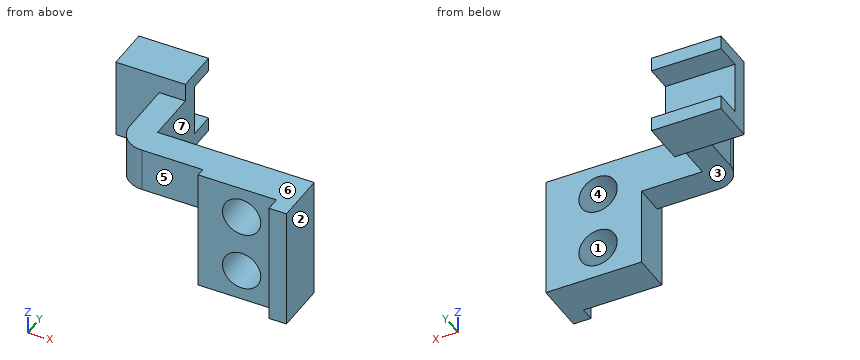
Autodesk Inventor part; units mm, degrees
ref_plane "YZ Plane" through (0, 0, 0) normal (1, 0, 0) x (0, 1, 0)
ref_plane "XZ Plane" through (0, 0, 0) normal (0, 1, 0) x (-1, 0, 0)
ref_plane "XY Plane" through (0, 0, 0) normal (0, 0, 1) x (1, 0, 0)
sketch "Sketch1" plane through (0, 0, 0) normal (0, 0, 1) x (1, 0, 0)
  line L0 (0, 0) -> (-100, 0)
  line L1 (-100, 0) -> (-100, 80)
  line L2 (-100, 80) -> (-550, 80)
  line L3 (-550, 80) -> (-550, 130)
  line L4 (-550, 130) -> (-1050, 130)
  line L5 (-1050, 130) -> (-1050, 600)
  line L6 (-1050, 600) -> (-900, 600)
  line L7 (-900, 600) -> (-900, 300)
  line L8 (-900, 300) -> (0, 300)
  line L9 (0, 300) -> (0, 0)
  line L10 (-550, 130) -> (-550, 300)
  dimension "d0" = 100
  dimension "d1" = 80
  dimension "d2" = 450
  dimension "d3" = 50
  dimension "d4" = 500
  dimension "d5" = 470
  dimension "d6" = 150
  dimension "d7" = 300
extrude "Extrusion1" add sketch "Sketch1" against normal blind 700 contours L0 L1 L2 L3 L10 L8 L9
sketch "Sketch2" plane through (0, 0, 0) normal (0, 0, 1) x (1, 0, 0)
  line L0 (-100, 80) -> (-550, 80) construction
  line L1 (-550, 80) -> (-550, 130)
  line L2 (-550, 80) -> (-550, 300) construction
  line L3 (-550, 130) -> (-1050, 130)
  line L4 (-1050, 130) -> (-1050, 600)
  line L5 (-1050, 600) -> (-900, 600)
  line L6 (-900, 600) -> (-900, 300)
  line L7 (-900, 300) -> (-550, 300)
  line L8 (-550, 300) -> (-550, 80) construction
  line L9 (-550, 130) -> (-550, 300)
  point P0 (0, 0)
  dimension "d10" = 50
  dimension "d11" = 500
  dimension "d12" = 470
  dimension "d13" = 150
  dimension "d14" = 300
extrude "Extrusion2" add sketch "Sketch2" against normal blind 250
sketch "Sketch3" plane through (-900, 300, 0) normal (1, 0, 0) x (0, 0, -1)
  line L0 (0, 300) -> (250, 300) construction
  line L1 (0, 300) -> (-105, 300)
  line L2 (-105, 300) -> (-105, 550)
  line L3 (-105, 550) -> (-25, 550)
  line L4 (-25, 550) -> (-25, 400)
  line L5 (-25, 400) -> (275, 400)
  line L6 (275, 400) -> (275, 550)
  line L7 (275, 550) -> (355, 550)
  line L8 (355, 550) -> (355, 300)
  line L9 (355, 300) -> (0, 300)
  point P0 (0, -300)
  dimension "d17" = 105
  dimension "d18" = 250
  dimension "d19" = 80
  dimension "d20" = 150
  dimension "d21" = 300
  dimension "d22" = 80
extrude "Extrusion3" add sketch "Sketch3" against normal blind 400
fillet "Fillet1" radius 150 1 edges at (-1050, 130, -125)
sketch "Sketch4" plane through (-550, 300, -700) normal (0, 1, 0) x (1, 0, 0)
  line L0 (450, -700) -> (550, -700) construction
  line L1 (550, -700) -> (550, -520)
  line L2 (550, -520) -> (250, -520)
  line L3 (250, -520) -> (250, -180)
  circle A0 centre (250, -520) radius 110
  circle A1 centre (250, -180) radius 110
  dimension "d26" = 180
  dimension "d27" = 300
  dimension "d28" = 340
  dimension "d29" = 220
  dimension "d30" = 220
extrude "Extrusion4" cut sketch "Sketch4" against normal blind 449.2125
properties part number "051665019_14"
The model under review builds one solid part; all positions refer to its coordinate system, in mm. Face numbers are marked on the shaded views. A direction names the side the tool comes from. Round coordinates to 2 decimals unless told otherwise and drop trailing zeros. Write each loop counter-clockwise with the first axis right and the second up, starting at its lowest first coordinate (ties: lowest second). Pieces come first, ordered by that corner, then holes. Notation, with made-up numbers: (62.5, 23) - (75.5, 23) arc R8 ccw to (75.5, 38) - close; hole circle Ø6 at (-4.75, 55). An arc over 180 degrees is marked (long way). Answer as CSV lines item,"result". Start each with the question number.
(1) To check wall thickness, follow line 1 (Z direction, x = -300, y = 215); line 2 (Z direction, x = -376, y = 162); line 3 (X direction, y = 613.5, z = -77.5). State the ranges of each line that lie inside material, in increasing order.
(2) We need section D-D on z = -520. State the section outline as (x, y) points.
(3) Draft analysis for pull direction X (two halves, no side actions). For the marked faces 1, 2, 3 and 4, state which applies: pulls with the +X half, pulls with the -X half, needs draft (parallel to the pull), parting line crosses it, or undercut.
(4) For pin 1 Ø8 at (y, z) = (181.5, -357) entering from -X; pin 2 Ø4 at (x, z) = (-167.5, -205.5) entering from -Y, all flat-tipped, find the tip position at first contact; note any pin that passes through.
(5) We need section C-C on y = 161. State the section outline as (x, z) points.
(6) We need section A-A on x = -300. State the section outline as (y, z) points.
(7) We need section B-B on z = -180. State the section outline as (x, y) points, plus the area to 3 significant figures.
(8) For the marked faces 5, 6 and 7, list the 3-axis set-ups (+Z, -Z, +X, -X, +Y, -Y) from which the entire face can be reached by the end or side of a thin tool; tool diameter is ignored.
Worked answers:
1,line 1,"-700 to -630, -410 to -290, -70 to 0"
1,line 2,"-700 to -599.52, -440.48 to -259.52, -100.48 to 0"
1,line 3,"-1300 to -900"
2,outline,"(-550, 80) - (-410, 80) - (-410, 300) - (-550, 300) - close; (-190, 80) - (-100, 80) - (-100, 0) - (0, 0) - (0, 300) - (-190, 300) - close"
3,face 1,"undercut"
3,face 2,"pulls with the +X half"
3,face 3,"needs draft"
3,face 4,"undercut"
4,pin 1,"x = -550"
4,pin 2,"y = 80"
5,outline,"(-991.32, -250) - (-550, -250) - (-550, -700) - (0, -700) - (0, 0) - (-991.32, 0) - close; hole circle Ø220 at (-300, -520); hole circle Ø220 at (-300, -180)"
6,outline,"(80, -700) - (300, -700) - (300, -630) - (80, -630) - close; (80, -410) - (300, -410) - (300, -290) - (80, -290) - close; (80, -70) - (300, -70) - (300, 0) - (80, 0) - close"
7,outline,"(-1300, 600) - (-1050, 600) - (-1050, 280) arc R150 ccw to (-900, 130) - (-550, 130) - (-550, 80) - (-410, 80) - (-410, 300) - (-900, 300) - (-900, 700) - (-1300, 700) - close; (-190, 80) - (-100, 80) - (-100, 0) - (0, 0) - (0, 300) - (-190, 300) - close"
7,area,"246,000 mm²"
8,face 5,"+Z, -Z, -X, -Y"
8,face 6,"+Z, +X, -X, -Y"
8,face 7,"+Z, -Z, +X, +Y"
